Check sheet for the drawn part. Datum: minimum x, y, z corner. Units: mm. Coordinates: 2 decimals unless noted, no trailing zeros. Write each loop counter-clockwise with the first axis right and the second up, starting at its lowest first coordinate (ties: lowest second). Pieces come first, ordered by that corner, then holes. Notation, with made-up numbers: M 23,79.25 L 47,79.25 A34 cw 47,116.25 Z; hole C 78.25,30 d6. An arc over 180 degrees is marked long. Write item = value, one per line. Start each with the question number.
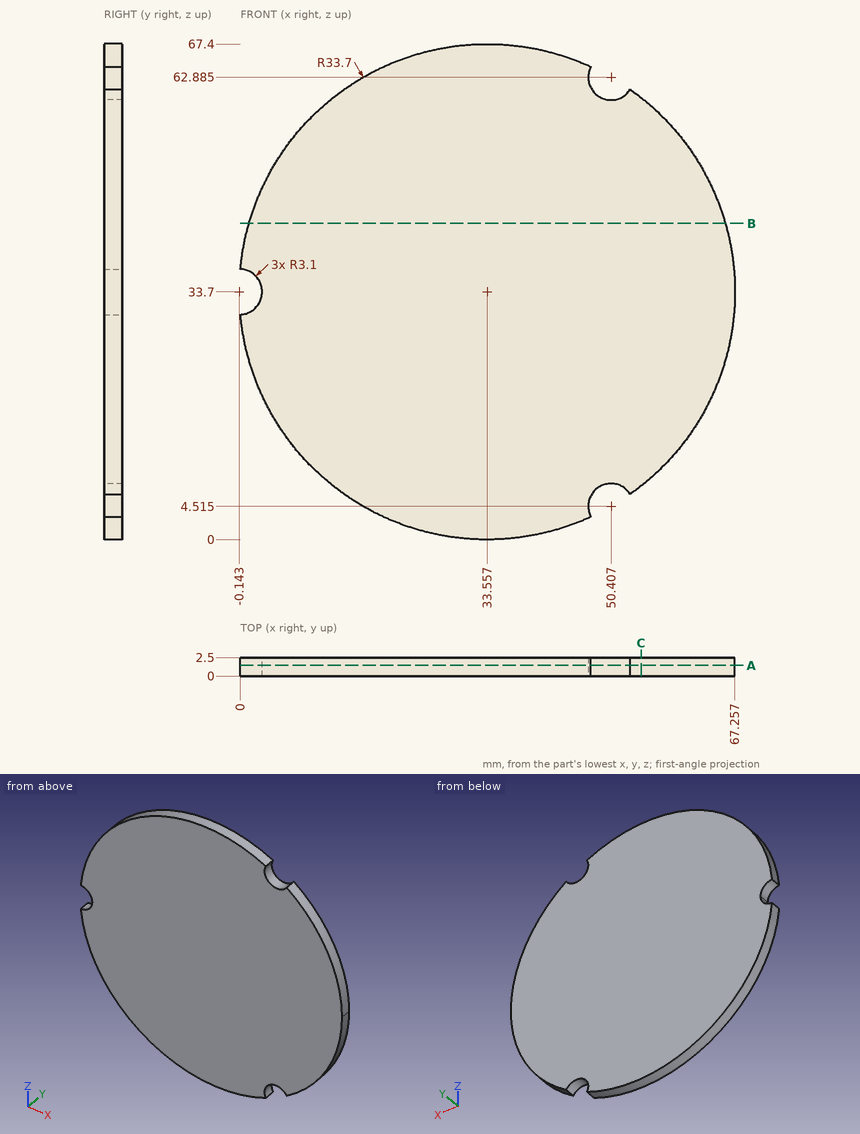
Q1. Scan lines: L1, parallel to Z at x = 33, y = 2 (1 decimal); L2, parallel to X at y = 2.1, z = 60.5 (1 decimal); L3, parallel to X at y = 1, z = 61 (1 decimal). Record each from-to range of solid material in increasing order.
Q2. Cross-section at C-C on x = 54.5. Enter the section's corners in (y, z).
Q3. Cross-section at B-B on z = 43. Enter the section's corners in (x, y).
Q4. Cross-section at A-A on y = 1.45. Enter the section's corners in (x, z) (1 decimal), and give its area (3 significant figures).
Q5. Gauge pin test, flat end, axial feed: pin 1 (1 mm diameter, centred on x = 39.5, y = 1, fed in from -Z). Record the tip position at first contact, or that the pin passes through.
Values found:
q1.L1 = 0 to 67.4
q1.L2 = 13.1 to 48.4, 52.4 to 54
q1.L3 = 13.8 to 47.9, 52.9 to 53.3
q2.outline = M 0,7.3 L 2.5,7.3 L 2.5,60.1 L 0,60.1 Z
q3.outline = M 1.17,0 L 65.95,0 L 65.95,2.5 L 1.17,2.5 Z
q4.outline = M 0,30.6 A33.7 ccw 47.7,3.1 A3.1 cw 53,6.2 A33.7 ccw 53,61.2 A3.1 cw 47.7,64.3 A33.7 ccw 0,36.8 A3.1 cw Z
q4.area = 3,520 mm²
q5.pin_1 = 0.44
